Geometry: final body of the model. Coordinates: model frame, mm. A direction names the side the tool comes from. Give positions to 0.01 mm unless a question says otherwise; leave off trailing zeros. Write each loop counter-clockwise with the first axis right and the second up, starting at its lowest first coordinate (ties: lowest second). Pieces come first, ordered by that corner, then holes.
```python
from build123d import *

# Parameters (mm, degrees)
IZIM1_R                           = 25
IZIM1_R_2                         = 17
Y_KSEKLIK_EKSTR_ZYON1_DEPTH       = 14
Y_KSEKLIK_EKSTR_ZYON2_DEPTH       = 14
IZIM2_W                           = 7
IZIM2_H                           = 16
Y_KSEKLIK_EKSTR_ZYON3_DEPTH       = 4
IZIM2_3_R                         = 6
Y_KSEKLIK_EKSTR_ZYON4_DEPTH       = 10
IZIM4_W                           = 7
IZIM4_H                           = 16
Y_KSEKLIK_EKSTR_ZYON11_DEPTH      = 10
Y_KSEKLIK_EKSTR_ZYON11_DEPTH_BACK = 4
Y_KSEKLIK_EKSTR_ZYON12_DEPTH      = 3.5


with BuildPart() as part:
    # izim1 → Y_kseklik-Ekstr_zyon1 (new body)
    with BuildSketch(Plane.XY):
        with Locations((15, 25)):
            Circle(IZIM1_R)
        with Locations((15, 25)):
            Circle(IZIM1_R_2, mode=Mode.SUBTRACT)
    extrude(amount=Y_KSEKLIK_EKSTR_ZYON1_DEPTH)

    # izim1_3 → Y_kseklik-Ekstr_zyon2 (add)
    with BuildSketch(Plane.XY):
        with BuildLine():
            Line((0, 5), (0, 0))
            Line((0, 0), (15, 0))
            ThreePointArc((15, 0), (7.09430585, 1.282917549), (0, 5))
        make_face()
        with BuildLine():
            ThreePointArc((40, 25), (32.67766953, 7.32233047), (15, 0))
            Line((15, 0), (40, 0))
            Line((40, 0), (40, 25))
        make_face()
    extrude(amount=Y_KSEKLIK_EKSTR_ZYON2_DEPTH)



with BuildPart() as body_2:
    # izim2 → Y_kseklik-Ekstr_zyon3 (new body)
    with BuildSketch(Plane(origin=(-32, 0, 0), x_dir=(0, 0, -1), z_dir=(1, 0, 0))):
        with Locations((-7, 8)):
            Rectangle(IZIM2_W, IZIM2_H)
    extrude(amount=Y_KSEKLIK_EKSTR_ZYON3_DEPTH)

    # izim2_3 → Y_kseklik-Ekstr_zyon4 (add)
    with BuildSketch(Plane(origin=(-32, 0, 0), x_dir=(0, 0, -1), z_dir=(1, 0, 0))):
        with BuildLine():
            Line((-3.5, 20), (-23.5, 20))
            ThreePointArc((-23.5, 20), (-33.5, 10), (-23.5, 0))
            Line((-23.5, 0), (-10.5, 0))
            Line((-10.5, 0), (-10.5, 16))
            Line((-10.5, 16), (-3.5, 16))
            Line((-3.5, 16), (-3.5, 20))
        make_face()
        with Locations((-23.5, 10)):
            Circle(IZIM2_3_R, mode=Mode.SUBTRACT)
    extrude(amount=Y_KSEKLIK_EKSTR_ZYON4_DEPTH)

    # izim4 → Y_kseklik-Ekstr_zyon11 (add, two sides)
    with BuildSketch(Plane(origin=(-32, 0, 0), x_dir=(0, 0, -1), z_dir=(1, 0, 0))) as y_kseklik_ekstr_zyon11_sk:
        with Locations((-7, 8)):
            Rectangle(IZIM4_W, IZIM4_H)
    extrude(amount=Y_KSEKLIK_EKSTR_ZYON11_DEPTH)
    extrude(y_kseklik_ekstr_zyon11_sk.sketch, amount=-Y_KSEKLIK_EKSTR_ZYON11_DEPTH_BACK)


with BuildPart() as part_1:
    add(part.part)

    add(body_2.part)  # Y_kseklik-Ekstr_zyon12 merges body 2
    # izim3 → Y_kseklik-Ekstr_zyon12 (add, symmetric)
    with BuildSketch(Plane.XY.offset(7)):
        with BuildLine():
            Line((-32, 20), (-0.393483787, 44.698747597))
            ThreePointArc((-0.393483787, 44.698747597), (-9.998772057, 24.752218594), (0, 5))
            Line((0, 5), (0, 0))
            Line((0, 0), (-22, 0))
            Line((-22, 0), (-22, 20))
            Line((-22, 20), (-32, 20))
        make_face()
    extrude(amount=Y_KSEKLIK_EKSTR_ZYON12_DEPTH, both=True)


solid = part_1.part
```
Item 1: Section A-A, the plane z = 8. Return the cut outline in (x, y).
Found:
outline: (-36, 0) - (40, 0) - (40, 25) arc R25 ccw to (-0.39, 44.7) - (-32, 20) - (-32, 16) - (-36, 16) - close; hole circle Ø34 at (15, 25)
Item 2: Reachability of faces 4 (the face through (15, 50, 7)), 5 (the face through (-34, 8, 10.5)), 6 (the face through (0, 3, 2)), 7 (the face through (-22, 10, 17)), 8 (the face through (-34, 16, 7)) from +Z, -Z, +X, -X, +Y, -Y: full face, straight path, thin tool, end or side. Return the list, or none.
Found:
face 4: none
face 5: +Z, -X, +Y, -Y
face 6: -Z, -X, -Y
face 7: +Z, +Y, -Y
face 8: +Z, -Z, -X, +Y
Item 3: Pull-direction query (X, two-part tool) for faces 1 (the face through (-36, 8, 7)), 2 (the face through (11.315, 8.404, 6.902)), 3 (the face through (-27, 20, 17)); classes: +X half, -X half, draft (parallel to the pull), parting line (faces both ways), or undercut.
Found:
face 1: -X half
face 2: undercut
face 3: draft
Item 4: Section C-C, the plane y = 26. Return the cut outline in (x, z), plus the area to 3 significant figures.
Found:
outline: (-24.32, 3.5) - (-9.98, 3.5) - (-9.98, 0) - (-1.97, 0) - (-1.97, 14) - (-9.98, 14) - (-9.98, 10.5) - (-24.32, 10.5) - close; (31.97, 0) - (39.98, 0) - (39.98, 14) - (31.97, 14) - close
area: 325 mm2
Item 5: Line query: L1, parallel to Y at x = 15, z = 3.5; L2, parallel to Y at x = -26.5, z = 23.5; L3, parallel to Z at x = 16, y = 5. Output: solid intervals per line, ascending.
Found:
L1: y = 0 to 8, 42 to 50
L2: y = 0 to 4, 16 to 20
L3: z = 0 to 14
Item 6: Section D-D, the plane y = 10. Return the cut outline in (x, z), plus the area to 3 significant figures.
Found:
outline: (-36, 3.5) - (-5, 3.5) - (-5, 0) - (7, 0) - (7, 14) - (-5, 14) - (-5, 10.5) - (-22, 10.5) - (-22, 17.5) - (-32, 17.5) - (-32, 10.5) - (-36, 10.5) - close; (-32, 29.5) - (-22, 29.5) - (-22, 33.5) - (-32, 33.5) - close; (23, 0) - (40, 0) - (40, 14) - (23, 14) - close
area: 733 mm2
Item 7: Pin query (flat end, axial travel): pin 1 Ø1.5 at (x, z) = (-27.5, 10.5) entering from +Y; pin 2 Ø5 at (y, z) = (17.5, 16.5) entering from -X; pin 3 Ø9.5 at (x, y) = (-12, 15.5) entering from +Z. Return the tip coordinate at first contact, or that it passes through.
Found:
pin 1: stops at y = 24.1
pin 2: stops at x = -32
pin 3: stops at z = 14
Item 8: Section B-B, the plane x = 15. Return the cut outline in (y, z), plus the area to 3 significant figures.
Found:
outline: (0, 0) - (8, 0) - (8, 14) - (0, 14) - close; (42, 0) - (50, 0) - (50, 14) - (42, 14) - close
area: 224 mm2
